```python
from build123d import *

# Parameters (mm, degrees)
F0_R     = 1.125
F0_R_2   = 3.25
F1_DEPTH = 3


with BuildPart() as f1:
    # F0 (on Top) → F1 (new body)
    with BuildSketch(Plane.XY):
        Polygon((-17, 0), (0, 0), (0, 7), (3, 7), (3, 17), (0, 17), (0, 24), (3, 24), (3, 34), (0, 34), (0, 41), (-17, 41), (-17, 44), (-27, 44), (-27, 41), (-36, 41), (-36, 35), (-35, 35), (-35, 33), (-36, 33), (-36, 30), (-38, 30), (-38, 33), (-39, 33), (-39, 35), (-38, 35), (-38, 41), (-47, 41), (-47, 44), (-57, 44), (-57, 41), (-66, 41), (-66, 35), (-65, 35), (-65, 33), (-66, 33), (-66, 30), (-68, 30), (-68, 33), (-69, 33), (-69, 35), (-68, 35), (-68, 41), (-77, 41), (-77, 44), (-87, 44), (-87, 41), (-104, 41), (-104, 34), (-107, 34), (-107, 24), (-104, 24), (-104, 17), (-107, 17), (-107, 7), (-104, 7), (-104, 0), (-87, 0), (-87, -3), (-77, -3), (-77, 0), (-68, 0), (-68, 6), (-69, 6), (-69, 8), (-68, 8), (-68, 11), (-66, 11), (-66, 8), (-65, 8), (-65, 6), (-66, 6), (-66, 0), (-57, 0), (-57, -3), (-47, -3), (-47, 0), (-38, 0), (-38, 6), (-39, 6), (-39, 8), (-38, 8), (-38, 11), (-36, 11), (-36, 8), (-35, 8), (-35, 6), (-36, 6), (-36, 0), (-27, 0), (-27, -3), (-17, -3), align=None)
        with Locations((-69.33824, 13.472463)):
            Circle(F0_R, mode=Mode.SUBTRACT)
        with Locations((-13.5, 19.8)):
            Circle(F0_R_2, mode=Mode.SUBTRACT)
        with Locations((-69.33824, 26.605537)):
            Circle(F0_R, mode=Mode.SUBTRACT)
    extrude(amount=F1_DEPTH)


solid = f1.part
```
Part model, mm, in its own coordinate system. A direction names the side the tool comes from. Round coordinates to 2 decimals unless told otherwise and drop trailing zeros. Write each loop counter-clockwise with the first axis right and the second up, starting at its lowest first coordinate (ties: lowest second). Pieces come first, ordered by that corner, then holes. Notation, with made-up numbers: M 5,8.25 L 64,8.25 A22 cw 64,24.25 Z; hole C 9.5,6.5 d7. An arc over 180 degrees is marked long. One line per question, with ' | ' between items.
(1) Saw through at B-B on x = -13.5. Write the cut outline in (y, z), then the cut area to 4 significant figures.
Answer key:
outline: M 0,0 L 16.55,0 L 16.55,3 L 0,3 Z; M 23.05,0 L 41,0 L 41,3 L 23.05,3 Z | area: 103.5 mm^2
(2) Pin check, flat tips, straight feed: pin 1 (1.5 mm diameter, centred on y = 42, z = 2, fed in from -X); pin 2 (2 mm diameter, centred on x = -62, y = 7, fed in from -Z); pin 3 (0.9 mm diameter, centred on y = 36.5, z = 1.5, fed in from -X); pin 4 (0.8 mm diameter, centred on x = -35.5, z = 2, fed in from -Y). Stop position of each tip, or through.
Answer key:
pin 1: stops at x = -87 | pin 2: stops at z = 0 | pin 3: stops at x = -104 | pin 4: stops at y = 0
(3) 3-axis set-ups, long thin cutter, end or side, ignore diameter. For faces 1 (the face through (-66, 38, 1)), 2 (the face through (1, 7, 1)), 3 (the face through (-87, -1, 1)), 4 (the face through (-73, 0, 1)): which of +Z, -Z, +X, -X, +Y, -Y reach the whole face in a straight line?
Answer key:
face 1: +Z, -Z, +Y | face 2: +Z, -Z, +X, -Y | face 3: +Z, -Z, -X, -Y | face 4: +Z, -Z, -Y
(4) Saw through at A-A on y = 19.8. Write the cut outline in (x, z), then the cut area to 4 significant figures.
Answer key:
outline: M -104,0 L -16.75,0 L -16.75,3 L -104,3 Z; M -10.25,0 L 0,0 L 0,3 L -10.25,3 Z | area: 292.5 mm^2
(5) Probe line 1 along X through (y, z) = (2, 2.05); line 2 along X through (y, z) = (8.5, 2.15); line 3 along Y through (x, z) = (-13.5, 2.1). List the from-to ranges inside material, lowest first.
Answer key:
line 1: x = -104 to -68, -66 to -38, -36 to 0 | line 2: x = -107 to -68, -66 to -38, -36 to 3 | line 3: y = 0 to 16.55, 23.05 to 41
(6) Two-plate mould, pull along Y, no slides. Class faces 5 (the face through (-107, 12, 1)), 6 (the face through (2, 17, 1)), 7 (the face through (-37, 30, 1)): released by +Y, released by -Y, zero draft, split by the parting line, or undercut.
Answer key:
face 5: zero draft | face 6: undercut | face 7: released by +Y
(7) Saw through at C-C on z = 0.45. Count the separate pieces of the cut face and the enclosed holes in it, then the cut area to 3 significant figures.
Answer key:
separate pieces: 1 | enclosed holes: 3 | area: 4,420 mm^2
